Can you work these out from the drawing? Everything is in mm from the part's minimum corner. A direction names the side the tool comes from. Coordinates: 2 decimals unless noted, no trailing zeros. Loops run counter-clockwise (first coordinate to the right, second up) from the corner with the lowest first, then second, coordinate; pieces in that order, holes last.
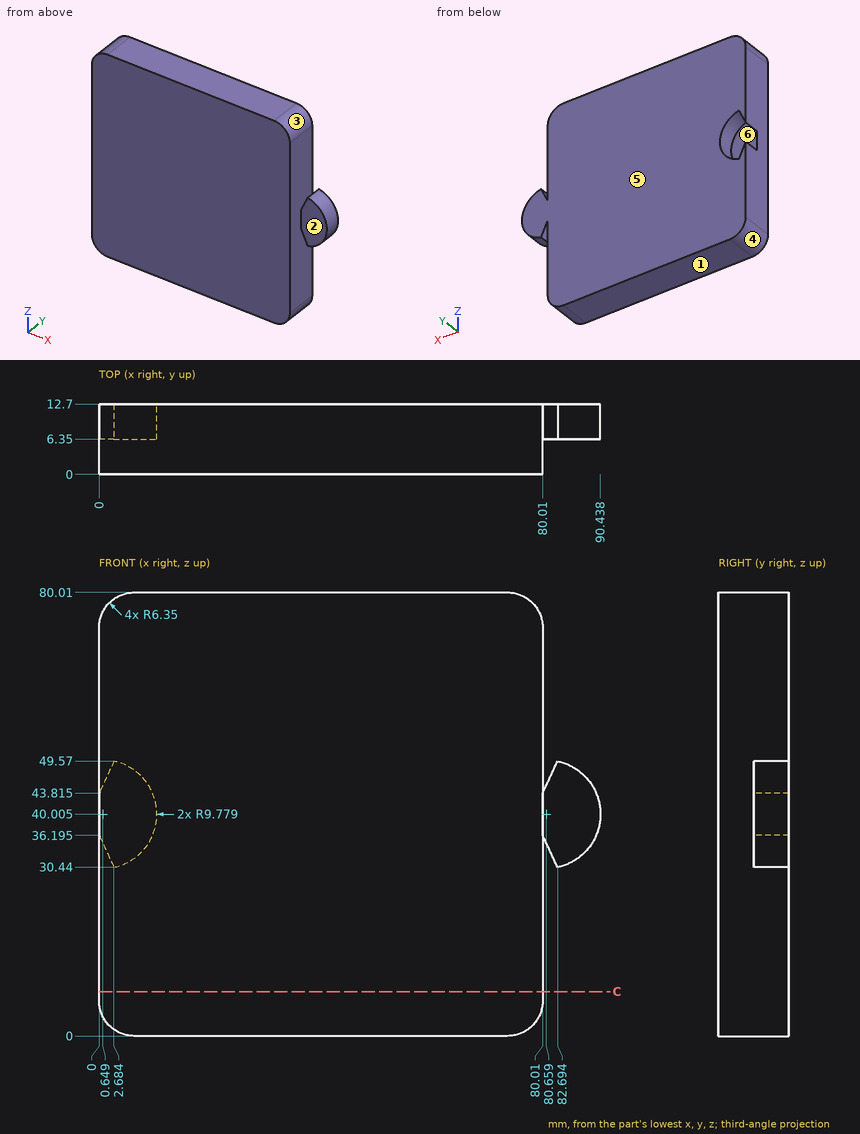
1) If I drill on L1, parallel to X at y = 11, z = 48; L2, parallel to X at y = 7.5, z = 35; L3, parallel to X at y = 3.25, z = 33, over which ranges is the centre line in solid material (lowest first)?
2) For the marked faces 1 and 2, which set-ups out of +Z, -Z, +X, -X, +Y, -Y let a thin tool reach every point of the face, with its end or its side?
3) Imagine slicing it at C-C on z = 8. List the corners of the cut face in (x, y) for me.
4) Will these pins go through, and if not, where does the flat tip stop? pin 1 (5 mm diameter, centred on x = 3, z = 41.5, fed in from +Y); pin 2 (8.5 mm diameter, centred on x = 84.5, z = 43.5, fed in from -Y).
5) We'd pull the mould along Z, two halves only. Please class the marked faces 3, 4, 5 and 6: released by +Z, released by -Z, zero draft, split by the parting line, or undercut.
Solved:
1. L1: x = 0 to 1.95, 6.28 to 80.01, 81.96 to 86.29
1. L2: x = 0 to 0.56, 9.05 to 80.01, 80.57 to 89.06
1. L3: x = 0 to 80.01
2. face 1: -Z, +X, -X, +Y, -Y
2. face 2: +Z, -Z, +X, -Y
3. outline: (0, 0) - (80.01, 0) - (80.01, 12.7) - (0, 12.7) - close
4. pin 1: stops at y = 6.35
4. pin 2: stops at y = 6.35
5. face 3: released by +Z
5. face 4: released by -Z
5. face 5: zero draft
5. face 6: undercut
